Here's how the part is built. I have some questions about the finished solid (model axes, mm). Face numbers are marked on the shaded views. A direction names the side the tool comes from. Round coordinates to 2 decimals unless told otherwise and drop trailing zeros. Loops run counter-clockwise (first coordinate to the right, second up) from the corner with the lowest first, then second, coordinate; pieces in that order, holes last. Notation, with made-up numbers: M -13,-38.75 L 18,-38.75 A28 cw 18,-5.75 Z; hole C 65,-9.75 d9. An arc over 180 degrees is marked long. Answer as a JSON object with one key per item and string values.
from build123d import *

# Parameters (mm, degrees)
BOSS_EXTRUDE1_DEPTH       = 30
CUT_EXTRUDE1_DEPTH        = 52.961524227
CUT_EXTRUDE1_DEPTH_BACK   = 52.961524227
SKETCH2_W                 = 46
SKETCH2_H                 = 46
FILLET1_R                 = 5
CHAMFER1_SIZE             = 1.75
M5X0_8_TAPPED_HOLE1_D     = 4.2
M5X0_8_TAPPED_HOLE1_DEPTH = 7
M5_CLEARANCE_HOLE1_D      = 5.5
M5_CLEARANCE_HOLE1_DEPTH  = 7
SKETCH11_R                = 12.5
CUT_EXTRUDE2_DEPTH        = 52.961524227
SKETCH12_R                = 20
CUT_EXTRUDE3_DEPTH        = 52.961524227


with BuildPart() as part:
    # Sketch1 → Boss-Extrude1 (new, symmetric)
    with BuildSketch(Plane(origin=(0, 0, 0), x_dir=(0, 0, -1), z_dir=(1, 0, 0))):
        Polygon((-30, -30), (-30, 30), (-23, 30), (-23, 15), (23, 15), (23, 30), (30, 30), (30, -30), (23, -30), (23, -15), (-23, -15), (-23, -30), align=None)
    extrude(amount=BOSS_EXTRUDE1_DEPTH, both=True)

    # Sketch2 → Cut-Extrude1 (cut, two sides: drawn at the far end of the back side and taken through both)
    with BuildSketch(Plane(origin=(0, 0, 0), x_dir=(1, 0, 0), z_dir=(0, 1, 0)).offset(-CUT_EXTRUDE1_DEPTH_BACK)):
        Rectangle(SKETCH2_W, SKETCH2_H)
    extrude(amount=CUT_EXTRUDE1_DEPTH + CUT_EXTRUDE1_DEPTH_BACK, mode=Mode.SUBTRACT)

    # Fillet1
    fillet1_edges = [part.edges().sort_by_distance(p)[0] for p in [
        (26.5, 15, -23),
        (26.5, -15, -23),
        (-26.5, 15, -23),
        (-26.5, -15, -23),
        (-23, 0, -23),
        (23, 0, -23),
    ]]
    fillet(fillet1_edges, radius=FILLET1_R)

    # Chamfer1
    chamfer1_edges = [part.edges().sort_by_distance(p)[0] for p in [
        (-30, 30, 26.5),
        (-30, 30, -26.5),
        (-30, -30, -26.5),
        (-30, -30, 26.5),
        (30, -30, -26.5),
        (30, 30, -26.5),
        (30, 30, 26.5),
        (30, -30, 26.5),
    ]]
    chamfer(chamfer1_edges, length=CHAMFER1_SIZE)

    # M5x0.8 Tapped Hole1
    with Locations(Plane(origin=(0, 0, -30), x_dir=(-1, 0, 0), z_dir=(0, 0, -1))):
        with Locations((-23.5, 23.5), (23.5, 23.5), (23.5, -23.5), (-23.5, -23.5)):
            Hole(M5X0_8_TAPPED_HOLE1_D / 2, depth=M5X0_8_TAPPED_HOLE1_DEPTH)

    # M5 Clearance Hole1
    with Locations(Plane.XY.offset(30)):
        with Locations((-13.5, 13.5), (-13.5, -13.5), (13.5, -13.5), (13.5, 13.5)):
            Hole(M5_CLEARANCE_HOLE1_D / 2, depth=M5_CLEARANCE_HOLE1_DEPTH)

    # Sketch11 → Cut-Extrude2 (cut, through all)
    with BuildSketch(Plane.XY):
        with Locations(Location((0, 0, 0), (0, 0, 270))):
            Circle(SKETCH11_R)
    extrude(amount=CUT_EXTRUDE2_DEPTH, mode=Mode.SUBTRACT)

    # Sketch12 → Cut-Extrude3 (cut, through all)
    with BuildSketch(Plane.XY):
        Circle(SKETCH12_R)
    extrude(amount=-CUT_EXTRUDE3_DEPTH, mode=Mode.SUBTRACT)


solid = part.part
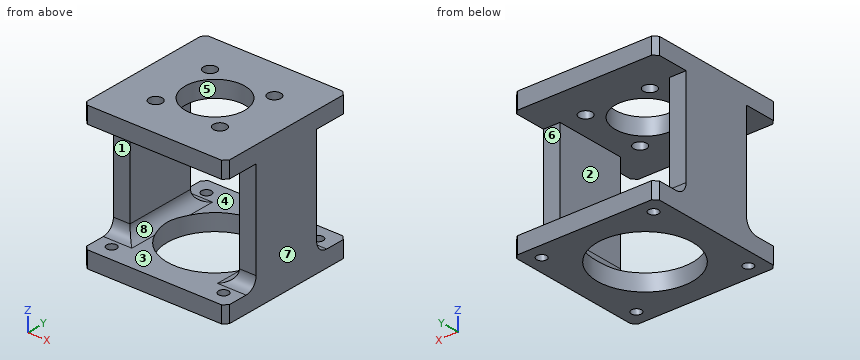
Item 1: I want a section at D-D, the plane z = 25. Please give me the cut outline in (x, y), then the cut area to 3 significant figures.
Resolved:
{"outline": "M -30,-28.25 L -28.25,-30 L 28.25,-30 L 30,-28.25 L 30,28.25 L 28.25,30 L -28.25,30 L -30,28.25 Z; hole C -13.5,-13.5 d5.5; hole C -13.5,13.5 d5.5; hole C 0,0 d25; hole C 13.5,-13.5 d5.5; hole C 13.5,13.5 d5.5", "area": "3,010 mm²"}
Item 2: I want a section at C-C, the plane y = -23.5. Please give me the cut outline in (x, z).
Resolved:
{"outline": "M -30,-30 L -25.6,-30 L -25.6,-23 L -30,-23 Z; M -30,23 L 30,23 L 30,30 L -30,30 Z; M -21.4,-30 L 21.4,-30 L 21.4,-23 L -21.4,-23 Z; M 25.6,-30 L 30,-30 L 30,-23 L 25.6,-23 Z"}
Item 3: Please list where these lines run through material, in increasing order: probe 1 along Y at (x, z) = (-23.5, -28.5); probe 2 along X at (y, z) = (-5, -8). Write a range as from..to.
Resolved:
{"probe 1": "-30..-25.6, -21.4..21.4, 25.6..30", "probe 2": "-30..-23, 23..30"}
Item 4: On a 3-axis mill with a long thin cutter (end or side, diameter ignored), from which of +Z, -Z, +X, -X, +Y, -Y can I reach the whole of each face in a straight line? I mean the marked faces 1, 2, 3 and 4. Say none if no direction works.
Resolved:
{"face 1": "+X, -X, -Y", "face 2": "+Y, -Y", "face 3": "-Y", "face 4": "+Y"}
Item 5: I want a section at A-A, the plane z = 0. Please give me the cut outline in (x, y), then the cut area to 3 significant figures.
Resolved:
{"outline": "M -30,-15 L -23,-15 L -23,15 L -30,15 Z; M 23,-15 L 30,-15 L 30,15 L 23,15 Z", "area": "420 mm²"}
Item 6: I'm going to push flat-ended pins straight in: pin 1 Ø8 at (x, y) = (15, -1) entering from -Z; pin 2 Ø2 at (x, z) = (-25, 3) entering from +Y; pin 3 Ø2 at (x, z) = (-26.5, 6.5) entering from -Y. Where does each tip first touch, or does it pass through?
Resolved:
{"pin 1": "z = 23", "pin 2": "y = 15", "pin 3": "y = -15"}
Item 7: If we mould it in two halves opening along X, with no side actions, what happens to the marked faces 5, 6, 7 and 8? For each: pulls with the +X half, pulls with the -X half, needs draft (parallel to the pull), parting line crosses it, or undercut.
Resolved:
{"face 5": "undercut", "face 6": "needs draft", "face 7": "pulls with the +X half", "face 8": "undercut"}
Item 8: I want a section at B-B, the plane y = 0. Please give me the cut outline in (x, z), then the cut area to 3 significant figures.
Resolved:
{"outline": "M -30,-30 L -20,-30 L -20,-22.58 A5 cw -23,-18 L -23,23 L -12.5,23 L -12.5,30 L -30,30 Z; M 12.5,23 L 23,23 L 23,-18 A5 cw 20,-22.58 L 20,-30 L 30,-30 L 30,30 L 12.5,30 Z", "area": "1,040 mm²"}
